The model under review builds one solid part; all positions refer to its coordinate system, in mm. A direction names the side the tool comes from. Round coordinates to 2 decimals unless told otherwise and drop trailing zeros. Order: outer loops, then holes, each group sorted by start corner. A loop starts at its lowest first (then second) coordinate and runs counter-clockwise, first axis right, second up.
from build123d import *

# Parameters (mm, degrees)
ESQUISSE1_R        = 40
BOSS_EXTRU_1_DEPTH = 200
BOSS_EXTRU_2_DEPTH = 25


with BuildPart() as part:
    # Esquisse1 → Boss.-Extru.1 (new body)
    with BuildSketch(Plane.XY):
        Circle(ESQUISSE1_R)
    extrude(amount=BOSS_EXTRU_1_DEPTH)

    # Esquisse2 → Boss.-Extru.2 (add)
    with BuildSketch(Plane.XY.offset(200)):
        Polygon((55.906189806, -14.416354416), (40.438024058, 41.208003393), (-15.468165749, 55.624357809), (-55.906189806, 14.416354416), (-40.438024058, -41.208003393), (15.468165749, -55.624357809), align=None)
    extrude(amount=BOSS_EXTRU_2_DEPTH)


solid = part.part
(1) We need section D-D (z = 173.5). Give the boundary of the cut face in (x, y), and give its area (3 significant figures).
(2) Tool access review of faces 1 (the flat face through (29, 29, 200)), 2 (the flat face through (-48.28, -13.01, 212.32)): name each direction out of +Z, -Z, +X, -X, +Y, -Y from which nothing blocks a thin tool from reaching the whole face with its end or side.
(3) We need section C-C (x = 0). Give the boundary of the cut face in (y, z).
(4) To check wall thickness, follow L1, parallel to Z at x = -50, y = 9; L2, parallel to Y at x = -1, z = 160; L3, parallel to Y at x = 23, z = 20.5. State the ranges of each line that lie inside material, in increasing order.
(5) Clearance check with flat-ended pins moving along their axes: P1, Ø6, axis at x = 6.5, z = 41.5, coming from the +Y side; P2, Ø3, axis at y = -34, z = 106.5, coming from the +X side; P3, Ø1, axis at y = -6, z = 63, coming from the -X side; P4, Ø3, axis at y = -42.5, z = 90, coming from the -X side. State where each tip first meets the part, or that it passes through.
(6) We need section B-B (y = -25). Give the boundary of the cut face in (x, z), and give its area (3 significant figures).
(7) The part is to be moulded in two halves that separate along Z. For faces 3 (the flat face through (-1, 1, 0)), 4 (the flat face through (12.876, 48.315, 212.325)), 5 (the flat face through (-1, 1, 225)), say which applies: pulls with the +Z half, pulls with the -Z half, needs draft (parallel to the pull), parting line crosses it, or undercut.
(8) We need section A-A (z = 207). Give the boundary of the cut face in (x, y).
Verdict:
1. outline: circle Ø80 at (0, 0)
1. area: 5,030 mm2
2. face 1: -Z
2. face 2: +Z, -Z, -X, -Y
3. outline: (-51.64, 200) - (-40, 200) - (-40, 0) - (40, 0) - (40, 200) - (51.64, 200) - (51.64, 225) - (-51.64, 225) - close
4. L1: z = 200 to 225
4. L2: y = -39.99 to 39.99
4. L3: y = -32.73 to 32.73
5. P1: stops at y = 39.85
5. P2: stops at x = 23.32
5. P3: stops at x = -39.62
5. P4: passes through
6. outline: (-44.95, 200) - (-31.22, 200) - (-31.22, 0) - (31.22, 0) - (31.22, 200) - (45.52, 200) - (45.52, 225) - (-44.95, 225) - close
6. area: 14,800 mm2
7. face 3: pulls with the -Z half
7. face 4: needs draft
7. face 5: pulls with the +Z half
8. outline: (-55.91, 14.42) - (-40.44, -41.21) - (15.47, -55.62) - (55.91, -14.42) - (40.44, 41.21) - (-15.47, 55.62) - close
